Autodesk Inventor part; units mm, degrees
ref_plane "YZ Plane" through (0, 0, 0) normal (1, 0, 0) x (0, 1, 0)
ref_plane "XZ Plane" through (0, 0, 0) normal (0, 1, 0) x (-1, 0, 0)
ref_plane "XY Plane" through (0, 0, 0) normal (0, 0, 1) x (1, 0, 0)
sketch "Sketch2" plane through (0, 0, 0) normal (0, 1, 0) x (-1, 0, 0)
  line L0 (15.1065, 12.5) -> (17.4159, 16.5)
  line L1 (17.4159, 16.5) -> (22.0347, 16.5)
  line L2 (22.0347, 16.5) -> (24.3441, 12.5)
  line L3 (24.3441, 12.5) -> (22.0347, 8.5)
  line L4 (22.0347, 8.5) -> (17.4159, 8.5)
  line L5 (17.4159, 8.5) -> (15.1065, 12.5)
  circle A0 centre (19.7253, 12.5) radius 2.55
  line L6 (13.6122, 19.5) -> (22.612, 19.5)
  line L7 (24.3441, 18.5) -> (26.7031, 14.414)
  line L8 (26.9711, 13.414) -> (26.9711, 0.8204)
  line L9 (13.6122, 19.5) -> (13.6603, 19.5)
  line L10 (0, 0) -> (8.2774, 0) construction
  line L11 (15.1065, -12.5) -> (17.4159, -16.5)
  line L12 (17.4159, -16.5) -> (22.0347, -16.5)
  line L13 (22.0347, -16.5) -> (24.3441, -12.5)
  line L14 (24.3441, -12.5) -> (22.0347, -8.5)
  line L15 (22.0347, -8.5) -> (17.4159, -8.5)
  line L16 (17.4159, -8.5) -> (15.1065, -12.5)
  circle A1 centre (19.7253, -12.5) radius 2.55
  line L17 (13.6603, -19.5) -> (22.612, -19.5)
  line L18 (24.3441, -18.5) -> (26.7031, -14.414)
  line L19 (26.9711, -13.414) -> (26.9711, -0.8204)
  line L20 (13.6122, -19.5) -> (13.6603, -19.5)
  line L21 (0, 25) -> (5, 25)
  line L22 (26.9711, 0.8204) -> (26.9711, -0.8204)
  line L23 (2, 20) -> (5, 20)
  line L24 (5, 20) -> (5, 25)
  line L25 (12.4782, 19.8526) -> (5, 25)
  arc A2 (12.4782, 19.8526) -> (13.6122, 19.5) centre (13.6122, 21.5) ccw
  arc A3 (24.3441, 18.5) -> (22.612, 19.5) centre (22.612, 17.5) ccw
  arc A4 (26.9711, 13.414) -> (26.7031, 14.414) centre (24.9711, 13.414) ccw
  line L26 (0, -25) -> (5, -25)
  line L27 (2, -20) -> (5, -20)
  line L28 (5, -20) -> (5, -25)
  line L29 (12.4782, -19.8526) -> (5, -25)
  arc A5 (13.6122, -19.5) -> (12.4782, -19.8526) centre (13.6122, -21.5) ccw
  arc A6 (22.612, -19.5) -> (24.3441, -18.5) centre (22.612, -17.5) ccw
  arc A7 (26.7031, -14.414) -> (26.9711, -13.414) centre (24.9711, -13.414) ccw
  line L30 (0, -25) -> (-1.0289, -25)
  line L31 (-1.0289, -25) -> (-1.0289, 25)
  line L32 (-1.0289, 25) -> (0, 25)
  line L33 (2, 20) -> (-1.0289, 20)
  line L34 (2, -20) -> (-1.0289, -20)
  point P0 (3, 23.2679)
  point P1 (19.7253, 8.5)
  point P2 (19.7253, 16.5)
  point P3 (23.7667, 19.5)
  point P4 (26.9711, 13.9499)
  point P5 (23.1894, 14.5)
  point P6 (12.9904, 19.5)
  point P7 (19.7253, -8.5)
  point P8 (19.7253, -16.5)
  point P9 (23.7667, -19.5)
  point P10 (26.9711, -13.9499)
  point P11 (23.1894, -14.5)
  point P12 (12.9904, -19.5)
  point P13 (25.239, 0.1796)
  point P14 (25.239, -0.1796)
  dimension "d18" = 8
  dimension "d19" = 5.1
  dimension "d21" = 3
  dimension "d22" = 3
  dimension "d27" = 25
  dimension "d33" = 5
  dimension "d34" = 2
  dimension "d35" = 2
  dimension "d36" = 2
  dimension "d37" = 2
  dimension "d48" = 28
extrude "Extrusion2" add sketch "Sketch2" along normal blind 35 contours L24 L23 L33 L31 L32 L21
extrude "Extrusion4" add sketch "Sketch2" along normal blind 3 contours L0 L1 L2 L3 L4 L5 | L16 L15 L14 L13 L12 L11
extrude "Extrusion6" add sketch "Sketch2" along normal blind 5 contours L6 A3 L7 A4 L8 L22 L19 A7 L18 A6 L17 L20 A5 L29 L28 L27 L34 L31 L33 L23 L24 L25 A2
extrude "Extrusion7" add sketch "Sketch2" along normal blind 35 contours L34 L27 L28 L26 L30 L31
sketch "Sketch4" plane through (0, 35, 0) normal (0, 1, 0) x (1, 0, 0)
  line L0 (-5, -25) -> (1.0289, -25)
  line L1 (0, -25) -> (-8, -25)
  line L2 (-10, -23) -> (-10, -22)
  line L3 (-8, -20) -> (0, -20)
  line L4 (0, 0) -> (-6.9228, 0) construction
  line L5 (0, 25) -> (-8, 25)
  line L6 (-10, 23) -> (-10, 22)
  line L7 (-8, 20) -> (0, 20)
  arc A0 (-10, -23) -> (-8, -25) centre (-8, -23) ccw
  arc A1 (-8, -20) -> (-10, -22) centre (-8, -22) ccw
  arc A2 (-10, 22) -> (-8, 20) centre (-8, 22) ccw
  arc A3 (-8, 25) -> (-10, 23) centre (-8, 23) ccw
  line L8 (1.0289, -20) -> (-5, -20)
  line L9 (0, -20) -> (1.0289, -20)
  line L10 (1.0289, -20) -> (1.0289, -25)
  line L11 (0, -25) -> (1.0289, -25)
  line L12 (-5, 20) -> (1.0289, 20)
  line L13 (0, 20) -> (1.0289, 20)
  line L14 (1.0289, 20) -> (1.0289, 25)
  line L15 (1.0289, 25) -> (0, 25)
  point P0 (-10, -20)
  point P1 (-10, -25)
  point P2 (-10, 20)
  point P3 (-10, 25)
  dimension "d42" = 10
  dimension "d43" = 5
  dimension "d44" = 2
extrude "Extrusion8" add sketch "Sketch4" along normal blind 3
properties part number "soporte_pinzas"
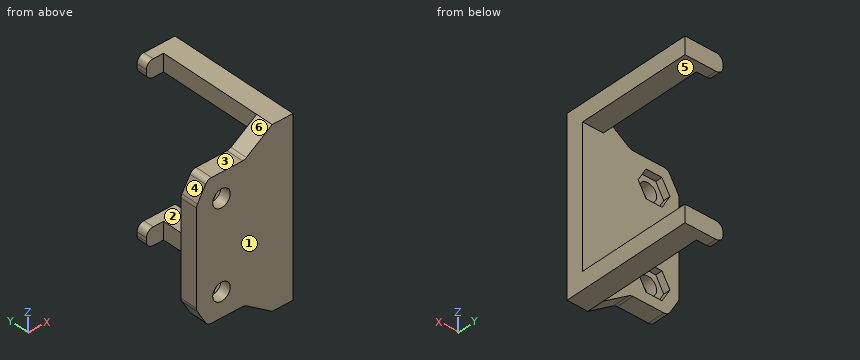
Read the model definition and answer for the solid it produces. Units are mm, in the model's axes. Face numbers are marked on the shaded views. A direction names the side the tool comes from. Give positions to 0.01 mm unless a question says otherwise; leave off trailing zeros. Loops run counter-clockwise (first coordinate to the right, second up) from the corner with the lowest first, then second, coordinate; pieces in that order, holes last. Notation, with made-up numbers: M 81,73 L 116,73 A4 cw 116,78 Z; hole C 37.25,2 d5. An arc over 180 degrees is marked long. Write each question's results on one line, items separated by ' | '.
1. The mould has two halves that part along Z. Classify the marked faces 1, 2 and 3: pulls with the +Z half, pulls with the -Z half, needs draft (parallel to the pull), parting line crosses it, or undercut.
Values:
face 1: needs draft | face 2: undercut | face 3: pulls with the +Z half
2. Straight lines are drawn through the part: line 1 (Z direction, x = -2, y = 12); line 2 (Y direction, x = -20, z = 6); line 3 (Y direction, x = -20.75, z = -15.5). For each, find the intervals that lie inside material, in ascending order. Write a range as [from, to].
Values:
line 1: z = [-25, -20], [20, 25] | line 2: y = [0, 5] | line 3: y = [0, 3]
3. Given pin 1 (4 mm diameter, centred on y = 15, z = -22.5, fed in from -X); pin 2 (2 mm diameter, centred on x = -20.5, y = 4.5, fed in from -Z); pin 3 (2 mm diameter, centred on x = -20.5, y = 4, fed in from +Z), each flat-ended and moving along its own axis, determine where each tip first touches the part or whether it passes through.
Values:
pin 1: stops at x = -5 | pin 2: stops at z = -19.5 | pin 3: stops at z = 19.5
4. Section C-C on x = -0.75 is taken. Give the vertices of the cut face in (y, z), plus the area to 3 significant figures.
Values:
outline: M 0,-25 L 38,-25 L 38,-20 L 5,-20 L 5,20 L 38,20 L 38,25 L 0,25 Z | area: 580 mm^2
5. Section A-A on y = 22 is taken. Give the vertices of the cut face in (x, z), plus the area to 3 significant figures.
Values:
outline: M -5,-25 L 1.03,-25 L 1.03,-20 L -5,-20 Z; M -5,20 L 1.03,20 L 1.03,25 L -5,25 Z | area: 60.3 mm^2
6. Section B-B on x = -6 is taken. Give the vertices of the cut face in (y, z), plus the area to 3 significant figures.
Values:
outline: M 0,-24.31 L 5,-24.31 L 5,24.31 L 0,24.31 Z; M 35,-25 L 38,-25 L 38,-20 L 35,-20 Z; M 35,20 L 38,20 L 38,25 L 35,25 Z | area: 273 mm^2
7. A tool of negligible diameter and unlimited length cuts with its end or side. For the marked faces 4, 5 and 6, from which of +Z, -Z, +X, -X, +Y, -Y can it reach the whole face along a straight path? Write none if from no direction.
Values:
face 4: +Z, -X, +Y, -Y | face 5: +X, -X, +Y | face 6: +Z, -X, -Y
